```python
from build123d import *

# Parameters (mm, degrees)
EXTRUDE_1_DEPTH        = 208
HOLE_WIZARD_M101_D     = 8.5
HOLE_WIZARD_M101_DEPTH = 27.5
HOLE_WIZARD_M101_TIP   = 2.553657631
SKETCH_6_R             = 6
CUT_EXTRUDE_2_DEPTH    = 216.555097365
PATTERN_LINEAR_1_COUNT = 2
PATTERN_LINEAR_1_PITCH = 214


with BuildPart() as part:
    # Эскиз1 → Бобышка-Вытянуть1 (new, symmetric)
    with BuildSketch(Plane.XY):
        with BuildLine():
            Line((-35, -20), (35, -20))
            ThreePointArc((35, -20), (38.535533906, -18.535533906), (40, -15))
            Line((40, -15), (40, 15))
            ThreePointArc((40, 15), (38.535533906, 18.535533906), (35, 20))
            Line((35, 20), (-35, 20))
            ThreePointArc((-35, 20), (-38.535533906, 18.535533906), (-40, 15))
            Line((-40, 15), (-40, -15))
            ThreePointArc((-40, -15), (-38.535533906, -18.535533906), (-35, -20))
        make_face()
        with BuildLine():
            Line((-35, -17), (35, -17))
            ThreePointArc((35, -17), (36.414213562, -16.414213562), (37, -15))
            Line((37, -15), (37, 15))
            ThreePointArc((37, 15), (36.414213562, 16.414213562), (35, 17))
            Line((35, 17), (-35, 17))
            ThreePointArc((-35, 17), (-36.414213562, 16.414213562), (-37, 15))
            Line((-37, 15), (-37, -15))
            ThreePointArc((-37, -15), (-36.414213562, -16.414213562), (-35, -17))
        make_face(mode=Mode.SUBTRACT)
    extrude(amount=EXTRUDE_1_DEPTH, both=True)

    # Отверстие обработанное метчиком M101
    with Locations(Plane(origin=(40, 0, 0), x_dir=(0, 0, -1), z_dir=(1, 0, 0))):
        with Locations((400, 3), (0, 3), (-400, 3)):
            Hole(HOLE_WIZARD_M101_D / 2, depth=HOLE_WIZARD_M101_DEPTH)
            with Locations((0, 0, -(HOLE_WIZARD_M101_DEPTH + HOLE_WIZARD_M101_TIP / 2))):  # 118° drill point
                Cone(0, HOLE_WIZARD_M101_D / 2, HOLE_WIZARD_M101_TIP, mode=Mode.SUBTRACT)

    # Эскиз6 → Вырез-Вытянуть2 (cut, symmetric)
    with BuildSketch(Plane.XZ.offset(20)):
        with Locations(Location((0, 132, 0), (0, 0, 270))):
            Circle(SKETCH_6_R)
        with Locations(Location((0, 82, 0), (0, 0, 270))):
            Circle(SKETCH_6_R)
    cut_extrude_2 = extrude(amount=CUT_EXTRUDE_2_DEPTH, both=True, mode=Mode.SUBTRACT)

    # Линейный массив1: Вырез-Вытянуть2 ×2
    with Locations(*[(0, 0, -i * PATTERN_LINEAR_1_PITCH) for i in range(1, PATTERN_LINEAR_1_COUNT)]):
        add(cut_extrude_2, mode=Mode.SUBTRACT)


solid = part.part
```
Design review of the part built by this model. Coordinates are the model's own, in mm. A direction names the side the tool comes from. Give positions to 0.01 mm unless a question says otherwise; leave off trailing zeros. Order: outer loops, then holes, each group sorted by start corner. A loop starts at its lowest first (then second) coordinate and runs counter-clockwise, first axis right, second up. Notation, with made-up numbers: M -28.5,34 L -15.5,34 A23 cw -15.5,42 Z; hole C -19,-26.5 d1. An arc over 180 degrees is marked long. One line per question, with ' | ' between items. Start each with the question number.
Q1. We need section A-A (y = 3). Write out the cut boundary in (x, z).
Q2. We need section C-C (x = 13.5). Write out the cut boundary in (y, z), plus the area to 3 significant figures.
Q3. The part is to be moulded in two halves that separate along X. For faces 4 (the face through (0, -19, -126)), 5 (the face through (-3, -18, 208)), 6 (the face through (40, -4, 3)), say which applies: +X half, -X half, draft (parallel to the pull), parting line (faces both ways), or undercut.
Q4. Machinability: for faces 1 (the face through (37, -4, 3)), 2 (the face through (-3.65, -18.52, -77.24)), 3 (the face through (38.479, 7.214, -0.553)), which of the approach directions +Z, -Z, +X, -X, +Y, -Y give a long, thin tool a straight path to every point of the face, cutting with its end or side? Answer none if there is none.
Q5. We need section B-B (z = 132). Write out the cut boundary in (x, y).
Q6. We need section D-D (z = 0). Write out the cut boundary in (x, y), plus the area to 3 significant figures.
Q7. For pin 1 Ø11 at (x, z) = (0, 132) entering from +Y, flat-tipped, find the tip position at first contact; note if it passes through.
Q8. For L1, parallel to Y at x = 20, z = 155.5; L2, parallel to X at y = 7, z = -156.5; L3, parallel to X at y = 18, z = 82, list the stretches that pass through material, from the lowest coordinate up. Write a range as [from, to].
Returned:
1) outline: M -40,-208 L -37,-208 L -37,208 L -40,208 Z; M 37,-208 L 40,-208 L 40,-4.25 L 37,-4.25 Z; M 37,4.25 L 40,4.25 L 40,208 L 37,208 Z
2) outline: M -20,-208 L -17,-208 L -17,208 L -20,208 Z; M 17,-208 L 20,-208 L 20,208 L 17,208 Z | area: 2,500 mm2
3) face 4: undercut | face 5: draft | face 6: +X half
4) face 1: +Z, -Z | face 2: +Y, -Y | face 3: +X
5) outline: M -40,-15 A5 ccw -35,-20 L -6,-20 L -6,-17 L -35,-17 A2 cw -37,-15 L -37,15 A2 cw -35,17 L -6,17 L -6,20 L -35,20 A5 ccw -40,15 Z; M 6,-20 L 35,-20 A5 ccw 40,-15 L 40,15 A5 ccw 35,20 L 6,20 L 6,17 L 35,17 A2 cw 37,15 L 37,-15 A2 cw 35,-17 L 6,-17 Z
6) outline: M -40,-15 A5 ccw -35,-20 L 35,-20 A5 ccw 40,-15 L 40,-1.25 L 37,-1.25 L 37,-15 A2 cw 35,-17 L -35,-17 A2 cw -37,-15 L -37,15 A2 cw -35,17 L 35,17 A2 cw 37,15 L 37,7.25 L 40,7.25 L 40,15 A5 ccw 35,20 L -35,20 A5 ccw -40,15 Z | area: 640 mm2
7) pin 1: through
8) L1: [-20, -17], [17, 20] | L2: [-40, -37], [37, 40] | L3: [-39, -6], [6, 39]
